```python
from build123d import *

# Parameters (mm, degrees)
CUT_EXTRUDE1_REACH = 33.75


with BuildPart() as part:
    # Sketch1 → Revolve1 (revolve)
    with BuildSketch(Plane.XY):
        Polygon((0, 31.75), (-2.38125, 31.75), (-3.175, 30.95625), (-3.175, 28.575), (-1.5875, 28.575), (-1.5875, 0.79375), (-0.79375, 0), (0, 0), align=None)
    revolve(axis=Axis((0, 0, 0), (0, 1, 0)))

    # Sketch2 → Cut-Extrude1 (cut, up to next)
    with BuildSketch(Plane(origin=(0, 31.75, 0), x_dir=(1, 0, 0), z_dir=(0, 1, 0)), mode=Mode.PRIVATE) as cut_extrude1_sk1:
        with BuildLine():
            Line((-2.749630657, 1.5875), (0, 3.175))
            ThreePointArc((0, 3.175), (-1.5875, 2.749630657), (-2.749630657, 1.5875))
        make_face()
    cut_extrude1_tool1 = extrude(cut_extrude1_sk1.sketch, amount=-CUT_EXTRUDE1_REACH, mode=Mode.PRIVATE) & part.part
    add(cut_extrude1_tool1.solids().sort_by_distance((-1.460397, 31.75, -2.529482))[0], mode=Mode.SUBTRACT)
    # Sketch2 → Cut-Extrude1 (cut, up to next)
    with BuildSketch(Plane(origin=(0, 31.75, 0), x_dir=(1, 0, 0), z_dir=(0, 1, 0)), mode=Mode.PRIVATE) as cut_extrude1_sk2:
        with BuildLine():
            ThreePointArc((2.749630657, 1.5875), (1.5875, 2.749630657), (0, 3.175))
            Line((0, 3.175), (2.749630657, 1.5875))
        make_face()
    cut_extrude1_tool2 = extrude(cut_extrude1_sk2.sketch, amount=-CUT_EXTRUDE1_REACH, mode=Mode.PRIVATE) & part.part
    add(cut_extrude1_tool2.solids().sort_by_distance((1.460397, 31.75, -2.529482))[0], mode=Mode.SUBTRACT)
    # Sketch2 → Cut-Extrude1 (cut, up to next)
    with BuildSketch(Plane(origin=(0, 31.75, 0), x_dir=(1, 0, 0), z_dir=(0, 1, 0)), mode=Mode.PRIVATE) as cut_extrude1_sk3:
        with BuildLine():
            ThreePointArc((3.175, 0), (3.066814498, 0.821750468), (2.749630657, 1.5875))
            Line((2.749630657, 1.5875), (2.749630657, -1.5875))
            ThreePointArc((2.749630657, -1.5875), (3.066814498, -0.821750468), (3.175, 0))
        make_face()
    cut_extrude1_tool3 = extrude(cut_extrude1_sk3.sketch, amount=-CUT_EXTRUDE1_REACH, mode=Mode.PRIVATE) & part.part
    add(cut_extrude1_tool3.solids().sort_by_distance((2.920795, 31.75, 0))[0], mode=Mode.SUBTRACT)
    # Sketch2 → Cut-Extrude1 (cut, up to next)
    with BuildSketch(Plane(origin=(0, 31.75, 0), x_dir=(1, 0, 0), z_dir=(0, 1, 0)), mode=Mode.PRIVATE) as cut_extrude1_sk4:
        with BuildLine():
            ThreePointArc((0, -3.175), (1.5875, -2.749630657), (2.749630657, -1.5875))
            Line((2.749630657, -1.5875), (0, -3.175))
        make_face()
    cut_extrude1_tool4 = extrude(cut_extrude1_sk4.sketch, amount=-CUT_EXTRUDE1_REACH, mode=Mode.PRIVATE) & part.part
    add(cut_extrude1_tool4.solids().sort_by_distance((1.460397, 31.75, 2.529482))[0], mode=Mode.SUBTRACT)
    # Sketch2 → Cut-Extrude1 (cut, up to next)
    with BuildSketch(Plane(origin=(0, 31.75, 0), x_dir=(1, 0, 0), z_dir=(0, 1, 0)), mode=Mode.PRIVATE) as cut_extrude1_sk5:
        with BuildLine():
            Line((0, -3.175), (-2.749630657, -1.5875))
            ThreePointArc((-2.749630657, -1.5875), (-1.5875, -2.749630657), (0, -3.175))
        make_face()
    cut_extrude1_tool5 = extrude(cut_extrude1_sk5.sketch, amount=-CUT_EXTRUDE1_REACH, mode=Mode.PRIVATE) & part.part
    add(cut_extrude1_tool5.solids().sort_by_distance((-1.460397, 31.75, 2.529482))[0], mode=Mode.SUBTRACT)
    # Sketch2 → Cut-Extrude1 (cut, up to next)
    with BuildSketch(Plane(origin=(0, 31.75, 0), x_dir=(1, 0, 0), z_dir=(0, 1, 0)), mode=Mode.PRIVATE) as cut_extrude1_sk6:
        with BuildLine():
            Line((-2.749630657, -1.5875), (-2.749630657, 1.5875))
            ThreePointArc((-2.749630657, 1.5875), (-3.175, 0), (-2.749630657, -1.5875))
        make_face()
    cut_extrude1_tool6 = extrude(cut_extrude1_sk6.sketch, amount=-CUT_EXTRUDE1_REACH, mode=Mode.PRIVATE) & part.part
    add(cut_extrude1_tool6.solids().sort_by_distance((-2.920795, 31.75, 0))[0], mode=Mode.SUBTRACT)


solid = part.part
```
Work out the finished part from the listing and answer in its coordinate system (mm). A direction names the side the tool comes from. Give positions to 0.01 mm unless a question says otherwise; leave off trailing zeros. Loops run counter-clockwise (first coordinate to the right, second up) from the corner with the lowest first, then second, coordinate; pieces in that order, holes last. Notation, with made-up numbers: M 14,80.25 L 34,80.25 A19 cw 34,87.25 Z; hole C 65.25,37 d3. An arc over 180 degrees is marked long. One line per item, written item: value. Start each with the question number.
1. Find section B-B (y = 29.5). Give the vertices of the cut face in (x, z) (1 decimal), and give its area (3 significant figures).
2. Each of these flat-tipped pins is pushed along its axis until it touches: P1, Ø1, axis at x = 1.5, y = 15.5, coming from the +Z side; P2, Ø3, axis at x = 0, y = 13, coming from the -Z side. Where does it stop, or does it pass through?
3. Which of the six approach directions +Z, -Z, +X, -X, +Y, -Y give full straight-line access (tool end or side, diameter ignored) to faces 1 (the face through (0.34, 14.49, -1.55)), 2 (the face through (1.36, 30, -2.39))?
4. Find the intervals of material crossed by probe 1 along Y at (x, z) = (-0.65, 1.75) (3 decimals); probe 2 along Z at (x, y) = (0.05, 21); probe 3 along Y at (x, z) = (-0.8, 2.25) (3 decimals), in increasing order.
5. Find section C-C (y = 13). Give the vertices of the cut face in (x, z) (1 decimal), and give its area (3 significant figures).
Reported:
1. outline: M -2.7,-1.6 L 0,-3.2 L 2.7,-1.6 L 2.7,1.6 L 0,3.2 L -2.7,1.6 Z
1. area: 26.2 mm²
2. P1: stops at z = 1.23
2. P2: stops at z = -1.59
3. face 1: -Y
3. face 2: -Z, +X, +Y, -Y
4. probe 1: y = 28.575 to 31.75
4. probe 2: z = -1.59 to 1.59
4. probe 3: y = 28.575 to 31.743
5. outline: C 0,0 d3.2
5. area: 7.92 mm²
